```python
from build123d import *

# Parameters (mm, degrees)
SKETCH_1_W          = 105
SKETCH_1_H          = 65.5
EXTRUDE_1_DEPTH     = 13
SHELL_1_T           = -2
SKETCH_2_R          = 3.5
SKETCH_2_R_2        = 6
SKETCH_2_W          = 15
SKETCH_2_H          = 10
CUT_EXTRUDE_1_DEPTH = 15
SKETCH_3_W          = 10.5
SKETCH_3_H          = 9
SKETCH_3_W_2        = 10
SKETCH_3_H_2        = 11
CUT_EXTRUDE_2_DEPTH = 15
CUT_EXTRUDE_3_DEPTH = 15
FILLET_1_R          = 2
SKETCH_5_W          = 2
SKETCH_5_H          = 17.199999525
CUT_EXTRUDE_4_DEPTH = 15
SKETCH_6_W          = 11
SKETCH_6_H          = 9
CUT_EXTRUDE_5_DEPTH = 15
SKETCH_10_W         = 2
SKETCH_10_H         = 15
SKETCH_10_W_2       = 15
SKETCH_10_H_2       = 2
EXTRUDE_2_DEPTH     = 25
FILLET_2_R          = 3
FILLET_3_R          = 5
SKETCH_11_R         = 1.4
CUT_EXTRUDE_6_DEPTH = 120
SKETCH_13_R         = 1.35
CUT_EXTRUDE_7_DEPTH = 76


with BuildPart() as part:
    # 草图1 → 凸台-拉伸1 (new body)
    with BuildSketch(Plane(origin=(0, 0, 0), x_dir=(1, 0, 0), z_dir=(0, 1, 0))):
        with Locations((0, 0.25)):
            Rectangle(SKETCH_1_W, SKETCH_1_H)
    extrude(amount=EXTRUDE_1_DEPTH)

    # 抽壳1
    shell_1_openings = [part.faces().sort_by_distance(p)[0] for p in [
        (0, 13, -0.25),
    ]]
    offset(amount=SHELL_1_T, openings=shell_1_openings, kind=Kind.INTERSECTION)

    # 草图2 → 切除-拉伸1 (cut)
    with BuildSketch(Plane.XY.offset(32.5)):
        with Locations((45.5, 13)):
            Circle(SKETCH_2_R)
        with Locations((31, 14)):
            Circle(SKETCH_2_R_2)
        with Locations((-40, 8)):
            Rectangle(SKETCH_2_W, SKETCH_2_H)
    extrude(amount=-CUT_EXTRUDE_1_DEPTH, mode=Mode.SUBTRACT)

    # 草图3 → 切除-拉伸2 (cut)
    with BuildSketch(Plane.ZY.offset(52.5)):
        with Locations((16.25, 8.5)):
            Rectangle(SKETCH_3_W, SKETCH_3_H)
        with Locations((-10.25, 8.5)):
            Rectangle(SKETCH_3_W, SKETCH_3_H)
        with Locations((3, 7.5)):
            Rectangle(SKETCH_3_W_2, SKETCH_3_H_2)
    extrude(amount=-CUT_EXTRUDE_2_DEPTH, mode=Mode.SUBTRACT)

    # 草图4 → 切除-拉伸3 (cut)
    with BuildSketch(Plane(origin=(52.5, 0, 0), x_dir=(0, 0, -1), z_dir=(1, 0, 0))):
        Polygon((31, 13), (14.225771641, 13), (12.965043457, 13), (-15.5, 13), (-15.5, 5), (12.965043457, 5), (14.225771641, 5), (14.225771641, 2.5), (31, 2.5), align=None)
    extrude(amount=-CUT_EXTRUDE_3_DEPTH, mode=Mode.SUBTRACT)

    # 圆角1
    fillet_1_edges = [part.edges().sort_by_distance(p)[0] for p in [
        (-52.5, 6.5, -33),
        (52.5, 6.5, -33),
        (52.5, 6.5, 32.5),
        (-52.5, 6.5, 32.5),
    ]]
    fillet(fillet_1_edges, radius=FILLET_1_R)

    # 草图5 → 切除-拉伸4 (cut)
    with BuildSketch(Plane(origin=(0, 0, -33), x_dir=(-1, 0, 0), z_dir=(0, 0, -1))):
        with Locations((-41.5, 10.748878275)):
            Rectangle(SKETCH_5_W, SKETCH_5_H)
        with Locations((-37.5, 10.748878275)):
            Rectangle(SKETCH_5_W, SKETCH_5_H)
        with Locations((-33.5, 10.748878275)):
            Rectangle(SKETCH_5_W, SKETCH_5_H)
        with Locations((-29.5, 10.748878275)):
            Rectangle(SKETCH_5_W, SKETCH_5_H)
        with Locations((-25.5, 10.748878275)):
            Rectangle(SKETCH_5_W, SKETCH_5_H)
        with Locations((-21.5, 10.748878275)):
            Rectangle(SKETCH_5_W, SKETCH_5_H)
    extrude(amount=-CUT_EXTRUDE_4_DEPTH, mode=Mode.SUBTRACT)

    # 草图6 → 切除-拉伸5 (cut)
    with BuildSketch(Plane(origin=(0, 0, -33), x_dir=(-1, 0, 0), z_dir=(0, 0, -1))):
        with Locations((41.5, 8.5)):
            Rectangle(SKETCH_6_W, SKETCH_6_H)
    extrude(amount=-CUT_EXTRUDE_5_DEPTH, mode=Mode.SUBTRACT)

    # 草图10 → 凸台-拉伸2 (add)
    with BuildSketch(Plane.XZ):
        with Locations((-53.5, -23.5)):
            Rectangle(SKETCH_10_W, SKETCH_10_H)
        with Locations((53.5, 23)):
            Rectangle(SKETCH_10_W, SKETCH_10_H)
        with Locations((13, -34)):
            Rectangle(SKETCH_10_W_2, SKETCH_10_H_2)
        with Locations((-23, 33.5)):
            Rectangle(SKETCH_10_W_2, SKETCH_10_H_2)
    extrude(amount=-EXTRUDE_2_DEPTH)

    # 圆角2
    # the kernel refuses this fillet: 3 mm, written as the material it adds along each edge
    with BuildSketch(Plane(origin=(52.5, 0, 30.5), x_dir=(-0.31622776601639135, 0, 0.9486832980506626), z_dir=(0, 1, 0)), Plane(origin=(-52.5, 0, -31), x_dir=(0.31622776601639135, 0, -0.9486832980506626), z_dir=(0, 1, 0))) as fillet_2_piece_1:
        with BuildLine():
            CenterArc((2.213594362, 2.846049894), FILLET_2_R, 198.434948823, 53.130102354)
            Line((-0.632455532, 1.897366596), (0, 0))
            ThreePointArc((0, 0), (0.632455532, 0.102633404), (1.264911064, 0))
        make_face()
    extrude(amount=13)
    with BuildSketch(Plane(origin=(-52.5, 0, -16), x_dir=(0, 0, 1), z_dir=(0, 1, 0))) as fillet_2_piece_2_section:
        with BuildLine():
            CenterArc((2.828427125, -3), FILLET_2_R, 90, 70.528779366)
            Line((0, -2), (0, 0))
            Line((0, 0), (2.828427125, 0))
        make_face()
    fillet_2_piece_2 = extrude(amount=20.071067812, mode=Mode.PRIVATE)
    fillet_2_piece_2 = split(fillet_2_piece_2, bisect_by=Plane(origin=(-52.5, 4, -16), z_dir=(0, -1, 0)), keep=Keep.TOP, mode=Mode.PRIVATE)
    add(fillet_2_piece_2)
    with BuildSketch(Plane(origin=(-52.5, -7.071067812, -16), x_dir=(0, 0, 1), z_dir=(0, 1, 0))) as fillet_2_piece_3_section:
        with BuildLine():
            CenterArc((2.828427125, -3), FILLET_2_R, 90, 70.528779366)
            Line((0, -2), (0, 0))
            Line((0, 0), (2.828427125, 0))
        make_face()
    fillet_2_piece_3 = extrude(amount=20.071067812, mode=Mode.PRIVATE)
    fillet_2_piece_3 = split(fillet_2_piece_3, bisect_by=Plane(origin=(-52.5, -7.071067812, -15.5), z_dir=(0, 0, -1)), keep=Keep.TOP, mode=Mode.PRIVATE)
    fillet_2_piece_3 = split(fillet_2_piece_3, bisect_by=Plane(origin=(-52.5, 4, -16), z_dir=(0, 1, 0)), keep=Keep.TOP, mode=Mode.PRIVATE)
    add(fillet_2_piece_3)
    with BuildSketch(Plane(origin=(52.5, 0, 15.5), x_dir=(0, 0, -1), z_dir=(0, 1, 0))) as fillet_2_piece_4:
        with BuildLine():
            CenterArc((2.828427125, -3), FILLET_2_R, 90, 70.528779366)
            Line((0, -2), (0, 0))
            Line((0, 0), (2.828427125, 0))
        make_face()
    extrude(amount=5)
    with BuildSketch(Plane(origin=(5.5, 0, -33), x_dir=(-1, 0, 0), z_dir=(0, 1, 0)), Plane(origin=(-15.5, 0, 32.5), x_dir=(1, 0, 0), z_dir=(0, 1, 0))) as fillet_2_piece_5:
        with BuildLine():
            CenterArc((2.828427125, -3), FILLET_2_R, 90, 70.528779366)
            Line((0, -2), (0, 0))
            Line((0, 0), (2.828427125, 0))
        make_face()
    extrude(amount=13)
    with BuildSketch(Plane(origin=(-30.5, 0, 32.5), x_dir=(-1, 0, 0), z_dir=(0, 1, 0))) as fillet_2_piece_6_section:
        with BuildLine():
            CenterArc((2.828427125, 3), FILLET_2_R, 199.471220634, 70.528779366)
            Line((0, 2), (0, 0))
            Line((0, 0), (2.828427125, 0))
        make_face()
    fillet_2_piece_6 = extrude(amount=20.071067812, mode=Mode.PRIVATE)
    fillet_2_piece_6 = split(fillet_2_piece_6, bisect_by=Plane(origin=(-30.5, 3, 32.5), z_dir=(0, -1, 0)), keep=Keep.TOP, mode=Mode.PRIVATE)
    add(fillet_2_piece_6)
    with BuildSketch(Plane(origin=(-30.5, -7.071067812, 32.5), x_dir=(-1, 0, 0), z_dir=(0, 1, 0))) as fillet_2_piece_7_section:
        with BuildLine():
            CenterArc((2.828427125, 3), FILLET_2_R, 199.471220634, 70.528779366)
            Line((0, 2), (0, 0))
            Line((0, 0), (2.828427125, 0))
        make_face()
    fillet_2_piece_7 = extrude(amount=20.071067812, mode=Mode.PRIVATE)
    fillet_2_piece_7 = split(fillet_2_piece_7, bisect_by=Plane(origin=(-30.5, 3, 32.5), z_dir=(0, 1, 0)), keep=Keep.TOP, mode=Mode.PRIVATE)
    fillet_2_piece_7 = split(fillet_2_piece_7, bisect_by=Plane(origin=(-32.5, -7.071067812, 32.5), z_dir=(1, 0, 0)), keep=Keep.TOP, mode=Mode.PRIVATE)
    add(fillet_2_piece_7)

    # 圆角3
    fillet_3_edges = [part.edges().sort_by_distance(p)[0] for p in [
        (-53.5, 25, -31),
        (-53.5, 25, -16),
        (53.5, 25, 30.5),
        (53.5, 25, 15.5),
        (20.5, 25, -34),
        (5.5, 25, -34),
        (-30.5, 25, 33.5),
        (-15.5, 25, 33.5),
    ]]
    fillet(fillet_3_edges, radius=FILLET_3_R)

    # 草图11 → 切除-拉伸6 (cut)
    with BuildSketch(Plane(origin=(54.5, 0, 0), x_dir=(0, 0, -1), z_dir=(1, 0, 0))):
        with Locations((-23, 20)):
            Circle(SKETCH_11_R)
        with Locations((23.5, 20)):
            Circle(SKETCH_11_R)
    extrude(amount=-CUT_EXTRUDE_6_DEPTH, mode=Mode.SUBTRACT)

    # 草图13 → 切除-拉伸7 (cut)
    with BuildSketch(Plane(origin=(0, 0, -35), x_dir=(-1, 0, 0), z_dir=(0, 0, -1))):
        with Locations((-13, 20)):
            Circle(SKETCH_13_R)
        with Locations((23, 20)):
            Circle(SKETCH_13_R)
    extrude(amount=-CUT_EXTRUDE_7_DEPTH, mode=Mode.SUBTRACT)


solid = part.part
```
Could you check a few things on this model? Use its own coordinates, in mm. A direction names the side the tool comes from. Give positions to 0.01 mm unless a question says otherwise; leave off trailing zeros. Loops run counter-clockwise (first coordinate to the right, second up) from the corner with the lowest first, then second, coordinate; pieces in that order, holes last. Notation, with made-up numbers: (74.25, 74) - (108.25, 74) arc R10 cw to (108.25, 93) - close; hole circle Ø6 at (-4.5, -37.75). An arc over 180 degrees is marked (long way). Use one line per item in the form item = value.
1. I want a section at B-B (z = 23). Please give me the cut outline in (x, y).
Response values:
outline = (-52.5, 0) - (54.5, 0) - (54.5, 18.6) - (52.5, 18.6) - (52.5, 13) - (50.5, 13) - (50.5, 2) - (-50.5, 2) - (-50.5, 13) - (-52.5, 13) - close; (52.5, 21.4) - (54.5, 21.4) - (54.5, 25) - (52.5, 25) - close
2. I want a section at D-D (x = 45.5). Please give me the cut outline in (y, z), and give its area (3 significant figures).
Response values:
outline = (0, -33) - (13, -33) - (13, -31) - (2, -31) - (2, 30.5) - (9.5, 30.5) - (9.5, 32.5) - (0, 32.5) - close
area = 168 mm²
3. On a 3-axis mill with a long thin cutter (end or side, diameter ignored), from which of +Z, -Z, +X, -X, +Y, -Y can I reach the whole of each face in a straight line? I mean faces 5 (the face through (5.5, 16, -34)), 6 (the face through (-52.5, 18, -24)), 7 (the face through (28.5, 7, -32)). Say none if no direction works.
Response values:
face_5 = +Z, -Z, -X, +Y
face_6 = +Z, -Z, +X, +Y
face_7 = -Z, +Y
4. Thinking about a two-plate mould opening in Z: for faces 1 (the face through (13, 12, -35)), 2 (the face through (52, 2.5, -22)), 3 (the face through (-52, 7, -2)), 4 (the face through (35, 13, -32)), which applies, released by +Z, released by -Z, zero draft, split by the parting line, or undercut?
Response values:
face_1 = released by -Z
face_2 = undercut
face_3 = undercut
face_4 = zero draft
5. I want a section at A-A (y = 15.75). Please give me the cut outline in (x, z), and give its area (3 significant figures).
Response values:
outline = (-54.5, -31) - (-52.5, -31) - (-52.5, -16) - (-54.5, -16) - close; (-30.5, 32.5) - (-15.5, 32.5) - (-15.5, 34.5) - (-30.5, 34.5) - close; (5.5, -35) - (20.5, -35) - (20.5, -33) - (5.5, -33) - close; (52.5, 15.5) - (54.5, 15.5) - (54.5, 30.5) - (52.5, 30.5) - close
area = 120 mm²
6. I need wall thicknesses on probe 1 along Z at (x, y) = (12, 11.75); probe 2 along Y at (x, z) = (53.4, 23); probe 3 along X at (y, z) = (8.5, 27). Which ranges of each line are inside material? Lowest first, please.
Response values:
probe_1 = -35 to -31, 30.5 to 32.5
probe_2 = 0 to 18.6, 21.4 to 25
probe_3 = -52.5 to -50.5, 50.5 to 54.5
7. I want a section at C-C (x = 13). Please give me the cut outline in (y, z), and give its area (3 significant figures).
Response values:
outline = (0, -35) - (18.65, -35) - (18.65, -33) - (13, -33) - (13, -31) - (2, -31) - (2, 30.5) - (13, 30.5) - (13, 32.5) - (0, 32.5) - close; (21.35, -35) - (25, -35) - (25, -33) - (21.35, -33) - close
area = 220 mm²
8. I'm going to push flat-ended pins straight in: pin 1 Ø1.6 at (x, z) = (27, -32) entering from +Y; pin 2 Ø2 at (y, z) = (3.5, -5.5) entering from +X; pin 3 Ø2.5 at (x, y) = (-51.5, 6.5) entering from +Z. Where does each tip first touch, or does it pass through?
Response values:
pin_1 = 13
pin_2 = 52.5
pin_3 = 32.5
